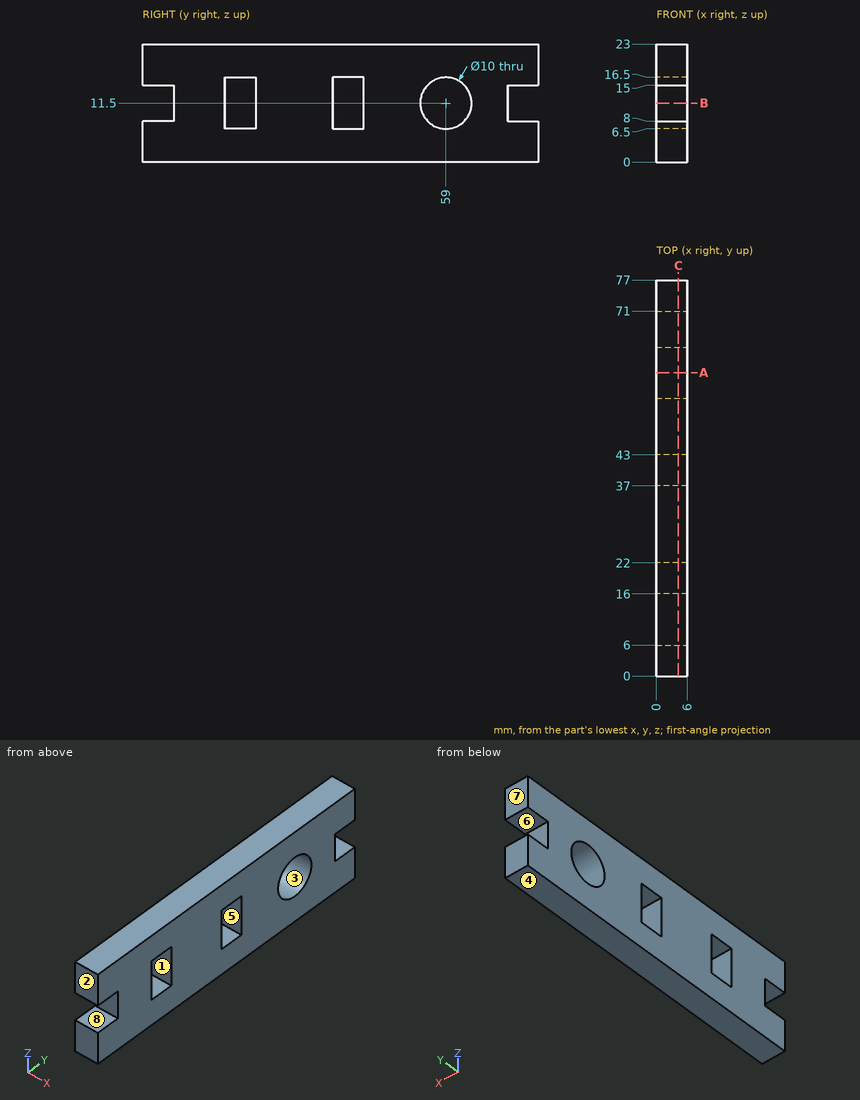
Part print with two shaded views. Sizes in mm from the minimum x, y, z corner. A direction names the side the tool comes from. Round coordinates to 2 decimals unless told otherwise and drop trailing zeros. Loops run counter-clockwise (first coordinate to the right, second up) from the corner with the lowest first, then second, coordinate; pieces in that order, holes last. Notation, with made-up numbers: M -29.75,52 L 18.25,52 A19 cw 18.25,77 Z; hole C -31,-2.5 d7. An arc over 180 degrees is marked long. Return JSON: item names as keys, results as strings. Group by question number.
(1) Tool access for the marked faces 5, 6, 7 and 8: list every direction of +Z, -Z, +X, -X, +Y, -Y with a clear straight run to the whole face (end or side of a thin tool).
(2) Wall check: probe 1 along Y at (x, z) = (2.2, 11.5); probe 2 along Z at (x, y) = (3.45, 74); probe 3 along Y at (x, z) = (2.15, 13). Give the ranges that are in metal, low to high. Write a range as [from, to].
(3) Saw through at C-C, the plane x = 4.25. List the corners of the cut face in (y, z), and give its area (3 significant figures).
(4) Saw through at B-B, the plane z = 11.5. List the corners of the cut face in (x, y).
(5) Drop flat-ended pins along their axis: P1, Ø1.8, axis at x = 1.5, z = 9.5, coming from the -Y side; P2, Ø1.8, axis at x = 2.5, z = 11, coming from the +Y side. Give the stop position or say it passes through.
(6) Saw through at A-A, the plane y = 59. List the corners of the cut face in (x, z), and give its area (3 significant figures).
(7) Mould opens along Y. For the marked faces 1, 2, 3 and 4 say: +Y half, -Y half, draft (parallel to the pull), parting line (faces both ways), or undercut.
Answer list:
{
 "1": {"face 5": "+X, -X", "face 6": "+X, -X, +Y", "face 7": "+Z, -Z, +X, -X, +Y", "face 8": "+X, -X, -Y"},
 "2": {"probe 1": "[6, 16], [22, 37], [43, 54], [64, 71]", "probe 2": "[0, 8], [15, 23]", "probe 3": "[6, 16], [22, 37], [43, 54.23], [63.77, 71]"},
 "3": {"outline": "M 0,0 L 77,0 L 77,8 L 71,8 L 71,15 L 77,15 L 77,23 L 0,23 L 0,15 L 6,15 L 6,8 L 0,8 Z; hole M 16,6.5 L 22,6.5 L 22,16.5 L 16,16.5 Z; hole M 37,6.5 L 43,6.5 L 43,16.5 L 37,16.5 Z; hole C 59,11.5 d10", "area": "1,490 mm2"},
 "4": {"outline": "M 0,6 L 6,6 L 6,16 L 0,16 Z; M 0,22 L 6,22 L 6,37 L 0,37 Z; M 0,43 L 6,43 L 6,54 L 0,54 Z; M 0,64 L 6,64 L 6,71 L 0,71 Z"},
 "5": {"P1": "y = 6", "P2": "y = 71"},
 "6": {"outline": "M 0,0 L 6,0 L 6,6.5 L 0,6.5 Z; M 0,16.5 L 6,16.5 L 6,23 L 0,23 Z", "area": "78.0 mm2"},
 "7": {"face 1": "undercut", "face 2": "-Y half", "face 3": "undercut", "face 4": "draft"}
}
